Model file for the job. Use its own axes, mm. A direction names the side the tool comes from. Round coordinates to 2 decimals unless told otherwise and drop trailing zeros. Write each loop counter-clockwise with the first axis right and the second up, starting at its lowest first coordinate (ties: lowest second). Pieces come first, ordered by that corner, then holes.
```python
from build123d import *

# Parameters (mm, degrees)
SKETCH_R       = 75
PAD_DEPTH      = 5
SKETCH001_R    = 25
PAD001_DEPTH   = 25
SKETCH002_R    = 22.5
POCKET_DEPTH   = 25
SKETCH003_W    = 12.2
SKETCH003_H    = 4.6
PAD002_DEPTH   = 17.2
CYLINDER_R     = 3
CYLINDER_DEPTH = 16


with BuildPart() as part:
    # Sketch → Pad (new body)
    with BuildSketch(Plane.XY):
        Circle(SKETCH_R)
    extrude(amount=PAD_DEPTH)

    # Sketch001 (on Face3 of Pad) → Pad001 (join)
    with BuildSketch(Plane.XY.offset(5)):
        Circle(SKETCH001_R)
    extrude(amount=PAD001_DEPTH)

    # Sketch002 (on Face5 of Pad001) → Pocket (cut)
    with BuildSketch(Plane.XY.offset(30)):
        Circle(SKETCH002_R)
    extrude(amount=-POCKET_DEPTH, mode=Mode.SUBTRACT)

    # Sketch003 (on Face7 of Pocket) → Pad002 (join)
    with BuildSketch(Plane.XY.offset(5)):
        with Locations((0, 13.9)):
            Rectangle(SKETCH003_W, SKETCH003_H)
        with Locations((0, -13.9)):
            Rectangle(SKETCH003_W, SKETCH003_H)
    extrude(amount=PAD002_DEPTH)

    # Cylinder → Cylinder (cut)
    with BuildSketch(Plane(origin=(0, -10.2, 8), x_dir=(1, 0, 0), z_dir=(0, -1, 0))):
        Circle(CYLINDER_R)
    extrude(amount=CYLINDER_DEPTH, mode=Mode.SUBTRACT)


solid = part.part
```
1) Cut at B-B on z = 8. List the corners of the cut face in (x, y), and give its area (3 significant figures).
2) Cut at A-A on y = 0. List the corners of the cut face in (x, z), and give its area (3 significant figures).
3) Pull direction Y, two halves, no side cores. Call faces 4 (the face through (-9.764, 74.362, 2.465)), 5 (the face through (-22.34, 3.82, 30)), 6 (the face through (0, -11.6, 13)): released by +Y, released by -Y, zero draft, split by the parting line, or undercut.
4) Which spindle directions (+Z, -Z, +X, -X, +Y, -Y) get a long thin tool onto all of the face, cutting with end or side? Do faces 1 (the face through (-6.1, -14, 13)), 2 (the face through (2.86, -23.63, 8.9)), 3 (the face through (-1, 1, 0)). Say none if no direction does.
5) Cut at C-C on x = 15. List the corners of the cut face in (y, z).
6) Cut at D-D on z = 25. List the corners of the cut face in (x, y), and give its area (3 significant figures).
7) Wall check: probe 1 along Z at (x, y) = (0, -23); probe 2 along X at (y, z) = (0, 20.5); probe 3 along Z at (x, y) = (-51.5, -36). Give the ranges that are in metal, low to high.
8) Flat gauge pins, fed straight in: pin 1 Ø10 at (x, z) = (2, 9.5) entering from +Y; pin 2 Ø3 at (y, z) = (-1.5, 23) entering from -X; pin 3 Ø2.5 at (y, z) = (14.5, 10.5) entering from -X. Where does each tip first touch, or does it go through?
Result sheet:
1. outline: (-6.1, -16.2) - (-3, -16.2) - (-3, -11.6) - (-6.1, -11.6) - close; (-6.1, 11.6) - (6.1, 11.6) - (6.1, 16.2) - (-6.1, 16.2) - close; (-3, -24.82) - (-3, -22.3) arc R22.5 cw (long way) to (3, -22.3) - (3, -24.82) arc R25 ccw (long way) to start; (3, -16.2) - (6.1, -16.2) - (6.1, -11.6) - (3, -11.6) - close
1. area: 443 mm2
2. outline: (-75, 0) - (75, 0) - (75, 5) - (25, 5) - (25, 30) - (22.5, 30) - (22.5, 5) - (-22.5, 5) - (-22.5, 30) - (-25, 30) - (-25, 5) - (-75, 5) - close
2. area: 875 mm2
3. face 4: split by the parting line
3. face 5: zero draft
3. face 6: undercut
4. face 1: +Z
4. face 2: -Y
4. face 3: -Z, +X, -X, +Y, -Y
5. outline: (-73.48, 0) - (73.48, 0) - (73.48, 5) - (20, 5) - (20, 30) - (16.77, 30) - (16.77, 5) - (-16.77, 5) - (-16.77, 30) - (-20, 30) - (-20, 5) - (-73.48, 5) - close
6. outline: circle Ø50 at (0, 0); hole circle Ø45 at (0, 0)
6. area: 373 mm2
7. probe 1: z = 0 to 5, 11 to 30
7. probe 2: x = -25 to -22.5, 22.5 to 25
7. probe 3: z = 0 to 5
8. pin 1: stops at y = 75
8. pin 2: stops at x = -25
8. pin 3: stops at x = -21.2
